from build123d import *

# Parameters (mm, degrees)
SKETCH_1_R               = 18
EXTRUDE_1_DEPTH          = 40
SKETCH_2_R               = 18.5
EXTRUDE_2_DEPTH          = 22.5
SKETCH_3_R               = 6
EXTRUDE_3_DEPTH          = 5
EXTRUDE_4_DEPTH          = 20
SKETCH_5_R               = 1.5
CUT_EXTRUDE_1_DEPTH      = 5
PATTERN_CIRCULAR_1_COUNT = 6


with BuildPart() as part:
    # 草图1 → 凸台-拉伸1 (new body)
    with BuildSketch(Plane.XY):
        Circle(SKETCH_1_R)
    extrude(amount=-EXTRUDE_1_DEPTH)

    # 草图2 → 凸台-拉伸2 (add)
    with BuildSketch(Plane.XY):
        with Locations(Location((0, 0, 0), (0, 0, 180))):
            Circle(SKETCH_2_R)
    extrude(amount=EXTRUDE_2_DEPTH)

    # 草图3 → 凸台-拉伸3 (add)
    with BuildSketch(Plane.XY.offset(22.5)):
        with Locations((-3.5, -6.062177826)):
            Circle(SKETCH_3_R)
    extrude(amount=EXTRUDE_3_DEPTH)

    # 草图4 → 凸台-拉伸4 (add)
    with BuildSketch(Plane.XY.offset(22.5)):
        with BuildLine():
            Line((-1.841687605, -3.562177826), (-5.158312395, -3.562177826))
            ThreePointArc((-5.158312395, -3.562177826), (-3.5, -9.062177826), (-1.841687605, -3.562177826))
        make_face()
    extrude(amount=EXTRUDE_4_DEPTH)

    # 草图5 → 切除-拉伸1 (cut)
    with BuildSketch(Plane.XY.offset(22.5)):
        with Locations((0, 15.5)):
            Circle(SKETCH_5_R)
    cut_extrude_1 = extrude(amount=-CUT_EXTRUDE_1_DEPTH, mode=Mode.SUBTRACT)

    # 阵列(圆周)1: 切除-拉伸1 ×6 about axis
    pattern_circular_1_axis = Axis((0, 0, 0), (0, 0, 1))
    for i in range(1, PATTERN_CIRCULAR_1_COUNT):
        add(cut_extrude_1.rotate(pattern_circular_1_axis, i * 360 / PATTERN_CIRCULAR_1_COUNT), mode=Mode.SUBTRACT)


solid = part.part
Source: CAD feature listing. Evaluate the final solid. Frame: model axes, mm. A direction names the side the tool comes from. Round coordinates to 2 decimals unless told otherwise and drop trailing zeros. Loops run counter-clockwise (first coordinate to the right, second up) from the corner with the lowest first, then second, coordinate; pieces in that order, holes last. Notation, with made-up numbers: (9.5, 35.25) -> (42.5, 35.25) arc R8 cw to (42.5, 45.25) -> close; hole circle Ø5 at (63.25, 71.5). An arc over 180 degrees is marked (long way). Answer as a JSON object with one key per item and string values. Group by question number.
Q1. Section query A-A (y = -5). Output: boundary loops of the cut face in (x, z).
Q2. Access query for faces 5 (the flat face through (-4, -3, 27.5)), 6 (the cylindrical face through (-2.343, 17.847, -19.72)), 7 (the flat face through (-3, -3.562, 35)). Directions: +Z, -Z, +X, -X, +Y, -Y. A direction counts if a zero-diameter tool reaches every point of the face in a straight line with its end or side. Return the directions, or none.
Q3. Section query D-D (x = 9.5). Output: boundary loops of the cut face in (y, z), plus the area to 3 significant figures.
Q4. Section query C-C (y = 7.75). Output: boundary loops of the cut face in (x, z), plus the area to 3 significant figures.
Q5. Contact query for flat-ended pins moving along their axis: P1, Ø2.5, axis at x = -13.42, y = 7.75, coming from the +Z side; P2, Ø3.5, axis at x = -0.5, y = 15.5, coming from the +Z side; P3, Ø3, axis at x = -10.5, z = 21.5, coming from the -Y side. Output: stop coordinate, or through.
Q6. Section query B-B (x = 0.5). Output: boundary loops of the cut face in (y, z).
Q7. Mould query, pull axis Y, two halves, no side actions, for faces 1 (the cylindrical face through (-7.922, -2.007, 24.965)), 2 (the flat face through (-13, -8, 17.5)), 3 (the flat face through (0, -16, 17.5)), 4 (the flat face through (-4.02, 17.73, 0)). Classes: pulls with the +Y half, pulls with the -Y half, needs draft (parallel to the pull), parting line crosses it, or undercut.
Q8. Ray query, line 1 (X direction, y = 7, z = 21); line 2 (Z direction, x = -6, y = 14); line 3 (Z direction, x = -12.5, y = 8). Return the intervals inside material, ascending. Write a range as from..to.
Completed:
{
 "1": {"outline": "(-17.81, 0) -> (-17.29, 0) -> (-17.29, -40) -> (17.29, -40) -> (17.29, 0) -> (17.81, 0) -> (17.81, 22.5) -> (2.41, 22.5) -> (2.41, 27.5) -> (-0.69, 27.5) -> (-0.69, 42.5) -> (-6.31, 42.5) -> (-6.31, 27.5) -> (-9.41, 27.5) -> (-9.41, 22.5) -> (-17.81, 22.5) -> close"},
 "2": {"face 5": "+Z", "face 6": "-Z", "face 7": "+Z, +X, -X, +Y"},
 "3": {"outline": "(-15.87, 0) -> (-15.29, 0) -> (-15.29, -40) -> (15.29, -40) -> (15.29, 0) -> (15.87, 0) -> (15.87, 22.5) -> (-15.87, 22.5) -> close", "area": "1,940 mm²"},
 "4": {"outline": "(-16.8, 0) -> (-16.25, 0) -> (-16.25, -40) -> (16.25, -40) -> (16.25, 0) -> (16.8, 0) -> (16.8, 22.5) -> (14.92, 22.5) -> (14.92, 17.5) -> (11.92, 17.5) -> (11.92, 22.5) -> (-11.92, 22.5) -> (-11.92, 17.5) -> (-14.92, 17.5) -> (-14.92, 22.5) -> (-16.8, 22.5) -> close", "area": "2,030 mm²"},
 "5": {"P1": "z = 17.5", "P2": "z = 22.5", "P3": "y = -16.16"},
 "6": {"outline": "(-18.49, 0) -> (-17.99, 0) -> (-17.99, -40) -> (17.99, -40) -> (17.99, 0) -> (18.49, 0) -> (18.49, 22.5) -> (16.91, 22.5) -> (16.91, 17.5) -> (14.09, 17.5) -> (14.09, 22.5) -> (-1.59, 22.5) -> (-1.59, 27.5) -> (-10.53, 27.5) -> (-10.53, 22.5) -> (-14.09, 22.5) -> (-14.09, 17.5) -> (-16.91, 17.5) -> (-16.91, 22.5) -> (-18.49, 22.5) -> close"},
 "7": {"face 1": "parting line crosses it", "face 2": "undercut", "face 3": "undercut", "face 4": "needs draft"},
 "8": {"line 1": "-17.12..-14.72, -12.12..12.12, 14.72..17.12", "line 2": "-40..22.5", "line 3": "-40..17.5"}
}
